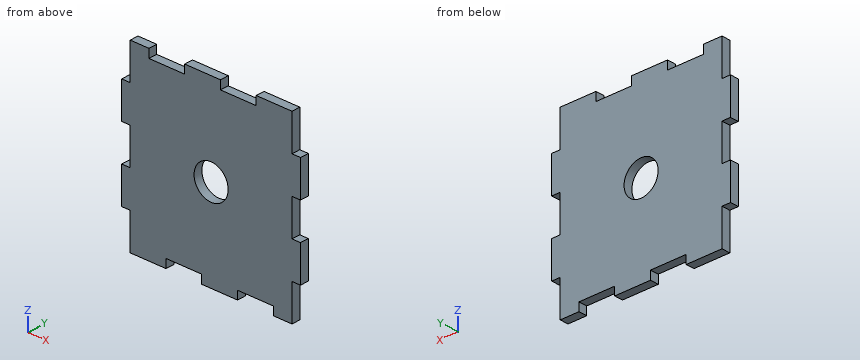
```python
from build123d import *

# Parameters (mm, degrees)
BOSS_EXTRUDE1_DEPTH = 4.7625
SKETCH3_R           = 9.525
CUT_EXTRUDE1_DEPTH  = 4.7625


with BuildPart() as part:
    # Sketch2 → Boss-Extrude1 (new body)
    with BuildSketch(Plane(origin=(0, 100, 0), x_dir=(1, 0, 0), z_dir=(0, 1, 0))):
        Polygon((80, 100), (80, 95.392875), (60, 95.392875), (60, 100), (40, 100), (40, 95.2375), (20, 95.2375), (20, 100), (0, 100), (0, 80), (-4.7625, 80), (-4.7625, 60), (0, 60), (0, 40), (-4.7625, 40), (-4.7625, 20), (0, 20), (0, 0), (10.475, 0), (10.475, 4.7625), (30.475, 4.7625), (30.475, 0), (50.475, 0), (50.475, 4.7625), (70.475, 4.7625), (70.475, 0), (90.475, 0), (90.475, 20), (95.2375, 20), (95.2375, 40), (90.475, 40), (90.475, 60), (95.2375, 60), (95.2375, 80), (90.475, 80), (90.475, 100), align=None)
    extrude(amount=-BOSS_EXTRUDE1_DEPTH)

    # Sketch3 → Cut-Extrude1 (cut)
    with BuildSketch(Plane(origin=(0, 100, 0), x_dir=(1, 0, 0), z_dir=(0, 1, 0))):
        with Locations(Location((45.2375, 50, 0), (0, 0, 270))):
            Circle(SKETCH3_R)
    extrude(amount=-CUT_EXTRUDE1_DEPTH, mode=Mode.SUBTRACT)


solid = part.part
```
Here's how the part is built. I have some questions about the finished solid (model axes, mm). Coordinates: 2 decimals unless noted, no trailing zeros. Loops run counter-clockwise (first coordinate to the right, second up) from the corner with the lowest first, then second, coordinate; pieces in that order, holes last. Notation, with made-up numbers: M 82,32.5 L 139,32.5 A23 ccw 139,59.5 Z; hole C 73.5,20.5 d5. An arc over 180 degrees is marked long. One line per item, written item: value.
1. Imagine slicing it at A-A (z = -50). List the corners of the cut face in (x, y) for me (1 decimal), and give its area (3 significant figures).
Geometry says:
outline: M 0,95.2 L 35.7,95.2 L 35.7,100 L 0,100 Z; M 54.8,95.2 L 90.5,95.2 L 90.5,100 L 54.8,100 Z
area: 340 mm2
2. Imagine slicing it at C-C (z = -93). List the corners of the cut face in (x, y) for me (1 decimal).
Geometry says:
outline: M 0,95.2 L 90.5,95.2 L 90.5,100 L 0,100 Z
3. Imagine slicing it at B-B (x = 68). List the corners of the cut face in (y, z) for me, and give its area (3 significant figures).
Geometry says:
outline: M 95.24,-95.39 L 100,-95.39 L 100,-4.76 L 95.24,-4.76 Z
area: 432 mm2
4. Please list where these lines run through material, in increasing order: probe 1 along X at (y, z) = (97.5, -50) (1 decimal); probe 2 along X at (y, z) = (96.2, -7) (3 decimals); probe 3 along Z at (x, y) = (16.5, 96).
Geometry says:
probe 1: x = 0 to 35.7, 54.8 to 90.5
probe 2: x = 0 to 90.475
probe 3: z = -100 to -4.76
5. Will these pins go through, and if not, where does the flat tip stop? pin 1 Ø2.5 at (y, z) = (97.5, -8.5) entering from -X; pin 2 Ø1.4 at (x, y) = (-3.5, 98) entering from +Z; pin 3 Ø2.5 at (x, y) = (61.5, 97) entering from +Z.
Geometry says:
pin 1: stops at x = 0
pin 2: stops at z = -20
pin 3: stops at z = -4.76
